For this review, take the finished solid that the model builds, in its own axes (mm). Face numbers are marked on the shaded views. A direction names the side the tool comes from. Coordinates: 2 decimals unless noted, no trailing zeros. Write each loop counter-clockwise with the first axis right and the second up, starting at its lowest first coordinate (ties: lowest second). Pieces come first, ordered by that corner, then holes.
```python
from build123d import *

# Parameters (mm, degrees)
SKETCH_1_W      = 14.3
SKETCH_1_H      = 12.2
SKETCH_1_R      = 0.875
SKETCH_1_R_2    = 0.907902719
EXTRUDE_1_DEPTH = 1.6
SKETCH_2_W      = 5.000412462
SKETCH_2_H      = 5.000412462
EXTRUDE_2_DEPTH = 1.6


with BuildPart() as part:
    # 草图1 → 凸台-拉伸1 (new body)
    with BuildSketch(Plane.XY):
        Rectangle(SKETCH_1_W, SKETCH_1_H)
        with Locations((2, 4.399857953)):
            Circle(SKETCH_1_R, mode=Mode.SUBTRACT)
        with Locations((2.05, -4.4)):
            Circle(SKETCH_1_R_2, mode=Mode.SUBTRACT)
    extrude(amount=EXTRUDE_1_DEPTH)

    # 草图2 → 凸台-拉伸2 (add)
    with BuildSketch(Plane(origin=(0, 0, 0), x_dir=(-1, 0, 0), z_dir=(0, 0, -1))):
        Rectangle(SKETCH_2_W, SKETCH_2_H)
    extrude(amount=EXTRUDE_2_DEPTH)


solid = part.part
```
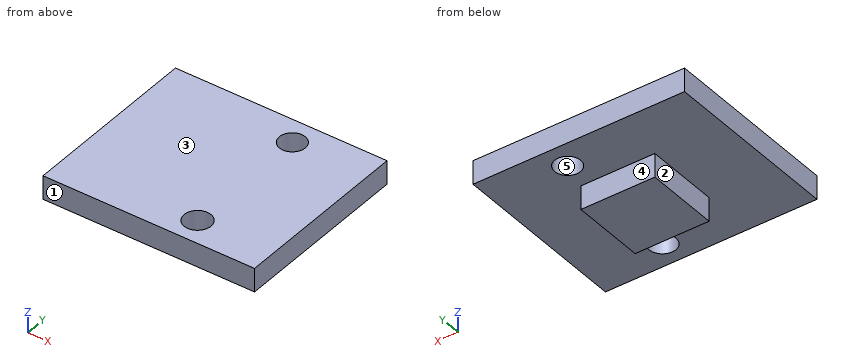
Q1. Add section B-B (x = 0). State the section outline as (y, z) points, then the cut area to 3 significant figures.
Ans:
outline: (-6.1, 0) - (-2.5, 0) - (-2.5, -1.6) - (2.5, -1.6) - (2.5, 0) - (6.1, 0) - (6.1, 1.6) - (-6.1, 1.6) - close
area: 27.5 mm2
Q2. Add section A-A (y = -4.4). State the section outline as (x, z) points, then the cut area to 3 significant figures.
Ans:
outline: (-7.15, 0) - (1.14, 0) - (1.14, 1.6) - (-7.15, 1.6) - close; (2.96, 0) - (7.15, 0) - (7.15, 1.6) - (2.96, 1.6) - close
area: 20.0 mm2
Q3. Add section D-D (z = 0.75). State the section outline as (x, y) points (3 decimals).
Ans:
outline: (-7.15, -6.1) - (7.15, -6.1) - (7.15, 6.1) - (-7.15, 6.1) - close; hole circle Ø1.75 at (2, 4.4); hole circle Ø1.816 at (2.05, -4.4)
Q4. For probe 1 along Y at (x, z) = (2, 0.95); probe 2 along Y at (x, z) = (1.5, 1); probe 3 along Z at (x, y) = (-6, 1), list the stretches that pass through material, from the lowest coordinate up.
Ans:
probe 1: y = -6.1 to -5.31, -3.49 to 3.52, 5.27 to 6.1
probe 2: y = -6.1 to -5.12, -3.68 to 3.68, 5.12 to 6.1
probe 3: z = 0 to 1.6
Q5. Clearance check with flat-ended pins moving along their axes: pin 1 Ø1.3 at (y, z) = (-1, -1) entering from -X; pin 2 Ø1 at (x, y) = (-3.5, 2.5) entering from -Z; pin 3 Ø0.5 at (y, z) = (1, -1) entering from +X. State where each tip first meets the part, or that it passes through.
Ans:
pin 1: stops at x = -2.5
pin 2: stops at z = 0
pin 3: stops at x = 2.5
Q6. Tool access review of the marked faces 1 and 2: name each direction out of +Z, -Z, +X, -X, +Y, -Y from which nothing blocks a thin tool from reaching the whole face with its end or side.
Ans:
face 1: +Z, -Z, +X, -X, -Y
face 2: -Z, -X, +Y, -Y
Q7. Draft analysis for pull direction Y (two halves, no side actions). For the marked faces 3, 4 and 5, state which applies: +Y half, -Y half, draft (parallel to the pull), parting line (faces both ways), or undercut.
Ans:
face 3: draft
face 4: +Y half
face 5: undercut
Q8. Add section C-C (x = 2). State the section outline as (y, z) points.
Ans:
outline: (-6.1, 0) - (-5.31, 0) - (-5.31, 1.6) - (-6.1, 1.6) - close; (-3.49, 0) - (-2.5, 0) - (-2.5, -1.6) - (2.5, -1.6) - (2.5, 0) - (3.52, 0) - (3.52, 1.6) - (-3.49, 1.6) - close; (5.27, 0) - (6.1, 0) - (6.1, 1.6) - (5.27, 1.6) - close
